```python
from build123d import *

# Parameters (mm, degrees)
F0_W     = 1790.7
F0_H     = 1694.18
F0_W_2   = 1536.7
F0_H_2   = 1440.18
F1_DEPTH = 485.14
F2_DEPTH = 25.4


with BuildPart() as f1:
    # F0 (on Top) → F1 (new body)
    with BuildSketch(Plane.XY):
        with Locations((768.35, 720.09)):
            Rectangle(F0_W, F0_H)
        with Locations((768.35, 720.09)):
            Rectangle(F0_W_2, F0_H_2, mode=Mode.SUBTRACT)
    extrude(amount=F1_DEPTH)

    # F0 (on Top) → F2 (join)
    with BuildSketch(Plane.XY):
        with Locations((768.35, 720.09)):
            Rectangle(F0_W, F0_H)
        with Locations((768.35, 720.09)):
            Rectangle(F0_W_2, F0_H_2, mode=Mode.SUBTRACT)
        with Locations((768.35, 720.09)):
            Rectangle(F0_W_2, F0_H_2)
    extrude(amount=-F2_DEPTH)


solid = f1.part
```
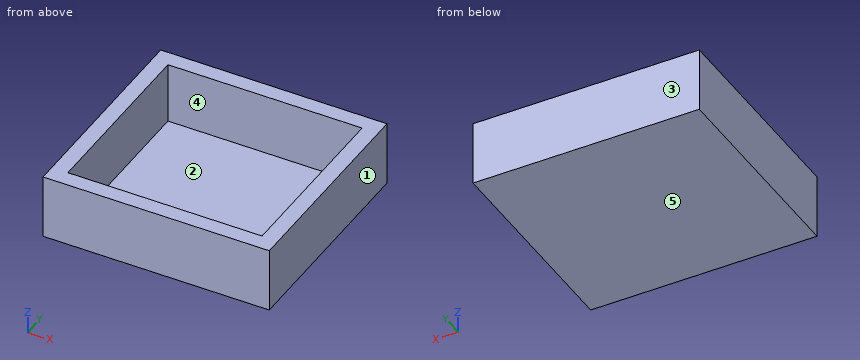
Check sheet for the modelled part. Datum: model origin and axes. Units: mm. Face numbers are marked on the shaded views. A direction names the side the tool comes from. Give positions to 0.01 mm unless a question says otherwise; leave off trailing zeros. Write each loop counter-clockwise with the first axis right and the second up, starting at its lowest first coordinate (ties: lowest second). Pieces come first, ordered by that corner, then holes.
Item 1: Access from +Z, -Z, +X, -X, +Y, -Y to the whole of each face (thin tool, end or side, straight path). Record for the marked faces 4 and 5.
Item 2: Cross-section at B-B (x = 954.5). Enter the section's corners in (y, z).
Item 3: Cross-section at C-C (y = 354). Enter the section's corners in (x, z), and give its area (3 significant figures).
Item 4: Gauge pin test, flat end, axial feed: pin 1 (1.5 mm diameter, centred on x = 868.5, y = 834.5, fed in from +Z). Record the tip position at first contact, or that the pin passes through.
Item 5: Cross-section at A-A (z = 158). Enter the section's corners in (x, y).
Item 6: Scan lines: L1, parallel to X at y = 551, z = 156.5; L2, parallel to Y at x = 231, z = 239; L3, parallel to Z at x = 126, y = 939.5. Record each from-to range of solid material in increasing order.
Item 7: Draft check along Y on the marked faces 1, 2 and 3. Enter one of: released by +Y, released by -Y, zero draft, split by the parting line, or undercut.
Report:
1. face 4: +Z
1. face 5: -Z, +X, -X, +Y, -Y
2. outline: (-127, -25.4) - (1567.18, -25.4) - (1567.18, 485.14) - (1440.18, 485.14) - (1440.18, 0) - (0, 0) - (0, 485.14) - (-127, 485.14) - close
3. outline: (-127, -25.4) - (1663.7, -25.4) - (1663.7, 485.14) - (1536.7, 485.14) - (1536.7, 0) - (0, 0) - (0, 485.14) - (-127, 485.14) - close
3. area: 169,000 mm2
4. pin 1: stops at z = 0
5. outline: (-127, -127) - (1663.7, -127) - (1663.7, 1567.18) - (-127, 1567.18) - close; hole (0, 0) - (1536.7, 0) - (1536.7, 1440.18) - (0, 1440.18) - close
6. L1: x = -127 to 0, 1536.7 to 1663.7
6. L2: y = -127 to 0, 1440.18 to 1567.18
6. L3: z = -25.4 to 0
7. face 1: zero draft
7. face 2: undercut
7. face 3: released by +Y
